Check sheet for the modelled part. Datum: model origin and axes. Units: mm. A direction names the side the tool comes from. Coordinates: 2 decimals unless noted, no trailing zeros. Write each loop counter-clockwise with the first axis right and the second up, starting at its lowest first coordinate (ties: lowest second). Pieces come first, ordered by that corner, then holes. Notation, with made-up numbers: (-11, 78) -> (22, 78) arc R27 cw to (22, 98) -> close; hole circle Ø9 at (80.5, -20). An arc over 180 degrees is marked (long way). One line per item, written item: value. Start each with the question number.
1) Set-up check for faces 1 (the flat face through (3, 98, -222.25)), 2 (the flat face through (3, 165, -90.5)), 3 (the flat face through (3, -4, -209.55)), 4 (the flat face through (3, 0, -251)): record each of +Z, -Z, +X, -X, +Y, -Y from which the full face is reachable in a straight line by a thin tool's end or side.
2) Sectioned sample at B-B on z = -106. Enter the section's corners in (x, y).
3) Scan lines: line 1 along Z through (x, y) = (1.35, 33) (3 decimals); line 2 along Z through (x, y) = (4.45, 175.5); line 3 along Z through (x, y) = (1.85, 20.5). Record each from-to range of solid material in increasing order. Write a range as [from, to].
4) Sectioned sample at C-C on y = 167.5. Enter the section's corners in (x, z).
5) Draft check along Y on faces 5 (the flat face through (3, -7.62, -105)), 6 (the flat face through (3, 31, 0)), 7 (the flat face through (3, 150, -85.471)). Enter one of: +Y half, -Y half, draft (parallel to the pull), parting line (faces both ways), or undercut.
6) Gauge pin test, flat ends, axial feed: P1, Ø1, axis at x = 0.5, z = -50, coming from the +Y side; P2, Ø2, axis at x = 2, z = -87, coming from the -Y side; P3, Ø3, axis at y = 142.5, z = -181.5, coming from the -X side. Record the tip position at first contact, or that the pin passes through.
7) Sectioned sample at A-A on y = 53. Enter the section's corners in (x, z) (3 decimals), plus the area to 3 significant figures.
8) Sectioned sample at D-D on x = 2.5. Give the number of separate pieces and of enclosed holes in the cut face, plus the area to 3 significant figures.
Autodesk Inventor part; units mm, degrees
ref_plane "YZ Plane" through (0, 0, 0) normal (1, 0, 0) x (0, 1, 0)
ref_plane "XZ Plane" through (0, 0, 0) normal (0, 1, 0) x (-1, 0, 0)
ref_plane "XY Plane" through (0, 0, 0) normal (0, 0, 1) x (1, 0, 0)
sketch "Sketch1" plane through (0, 0, 0) normal (1, 0, 0) x (0, 1, 0)
  line L0 (0, 0) -> (177.8, 0)
  line L1 (177.8, -260.35) -> (0, -260.35)
  line L2 (0, -260.35) -> (0, -241.3)
  line L3 (0, -241.3) -> (-7.62, -241.3)
  line L4 (-7.62, -241.3) -> (-7.62, -222.25)
  line L5 (-7.62, -222.25) -> (0, -222.25)
  line L6 (0, -209.55) -> (-7.62, -209.55)
  line L7 (-7.62, -209.55) -> (-7.62, -190.5)
  line L8 (-7.62, -190.5) -> (0, -190.5)
  line L9 (0, -190.5) -> (0, -152.4)
  line L10 (44.45, -215.9) -> (44.45, -214.2998)
  line L11 (44.45, -217.5002) -> (44.45, -215.9)
  line L12 (24.6348, -214.2998) -> (24.6348, -212.725)
  line L13 (24.6348, -219.075) -> (24.6348, -219.329)
  line L14 (24.6348, -219.329) -> (30.1625, -219.329)
  line L15 (24.6348, -212.725) -> (24.6348, -212.471)
  line L16 (24.6348, -212.471) -> (30.1625, -212.471)
  line L17 (24.6348, -219.075) -> (24.6348, -217.4875)
  line L18 (30.1625, -212.471) -> (30.1625, -214.2998)
  line L19 (30.1625, -217.5002) -> (30.1625, -219.329)
  line L20 (44.45, -214.2998) -> (30.1625, -214.2998)
  line L21 (24.6348, -214.2998) -> (0, -214.2998)
  line L22 (44.45, -217.5002) -> (30.1625, -217.5002)
  line L23 (24.6348, -217.5002) -> (0, -217.5002)
  line L24 (0, -63.5) -> (-7.62, -63.5)
  line L25 (-7.62, -63.5) -> (-7.62, -82.55)
  line L26 (-7.62, -82.55) -> (0, -82.55)
  line L27 (0, -95.25) -> (-7.62, -95.25)
  line L28 (-7.62, -95.25) -> (-7.62, -114.3)
  line L29 (-7.62, -114.3) -> (0, -114.3)
  line L30 (44.45, -88.9) -> (44.45, -90.5002)
  line L31 (44.45, -87.2998) -> (44.45, -88.9)
  line L32 (24.6348, -90.5002) -> (24.6348, -92.075)
  line L33 (24.6348, -85.725) -> (24.6348, -85.471)
  line L34 (24.6348, -85.471) -> (30.1625, -85.471)
  line L35 (24.6348, -92.075) -> (24.6348, -92.329)
  line L36 (24.6348, -92.329) -> (30.1625, -92.329)
  line L37 (24.6348, -85.725) -> (24.6348, -87.3125)
  line L38 (30.1625, -92.329) -> (30.1625, -90.5002)
  line L39 (30.1625, -87.2998) -> (30.1625, -85.471)
  line L40 (44.45, -90.5002) -> (30.1625, -90.5002)
  line L41 (24.6348, -90.5002) -> (0, -90.5002)
  line L42 (44.45, -87.2998) -> (30.1625, -87.2998)
  line L43 (24.6348, -87.2998) -> (0, -87.2998)
  line L44 (177.8, -241.3) -> (185.42, -241.3)
  line L45 (185.42, -241.3) -> (185.42, -222.25)
  line L46 (185.42, -222.25) -> (177.8, -222.25)
  line L47 (177.8, -209.55) -> (185.42, -209.55)
  line L48 (185.42, -209.55) -> (185.42, -190.5)
  line L49 (185.42, -190.5) -> (177.8, -190.5)
  line L50 (177.8, -190.5) -> (177.8, -152.4)
  line L51 (133.35, -215.9) -> (133.35, -214.2998)
  line L52 (133.35, -217.5002) -> (133.35, -215.9)
  line L53 (153.1652, -214.2998) -> (153.1652, -212.725)
  line L54 (153.1652, -219.075) -> (153.1652, -219.329)
  line L55 (153.1652, -219.329) -> (147.6375, -219.329)
  line L56 (153.1652, -212.725) -> (153.1652, -212.471)
  line L57 (153.1652, -212.471) -> (147.6375, -212.471)
  line L58 (153.1652, -219.075) -> (153.1652, -217.4875)
  line L59 (147.6375, -212.471) -> (147.6375, -214.2998)
  line L60 (147.6375, -217.5002) -> (147.6375, -219.329)
  line L61 (133.35, -214.2998) -> (147.6375, -214.2998)
  line L62 (153.1652, -214.2998) -> (177.8, -214.2998)
  line L63 (133.35, -217.5002) -> (147.6375, -217.5002)
  line L64 (153.1652, -217.5002) -> (177.8, -217.5002)
  line L65 (185.42, -63.5) -> (185.42, -82.55)
  line L66 (185.42, -82.55) -> (177.8, -82.55)
  line L67 (177.8, -95.25) -> (185.42, -95.25)
  line L68 (185.42, -95.25) -> (185.42, -114.3)
  line L69 (185.42, -114.3) -> (177.8, -114.3)
  line L70 (153.1652, -85.725) -> (153.1652, -85.471)
  line L71 (153.1652, -85.725) -> (153.1652, -87.3125)
  line L72 (153.1652, -85.471) -> (147.6375, -85.471)
  line L73 (147.6375, -87.2998) -> (147.6375, -85.471)
  line L74 (177.8, -63.5) -> (185.42, -63.5)
  line L75 (153.1652, -90.5002) -> (153.1652, -92.075)
  line L76 (153.1652, -92.075) -> (153.1652, -92.329)
  line L77 (153.1652, -92.329) -> (147.6375, -92.329)
  line L78 (147.6375, -92.329) -> (147.6375, -90.5002)
  line L79 (133.35, -87.2998) -> (147.6375, -87.2998)
  line L80 (133.35, -87.2998) -> (133.35, -88.9)
  line L81 (133.35, -90.5002) -> (147.6375, -90.5002)
  line L82 (153.1652, -87.2998) -> (177.8, -87.2998)
  line L83 (153.1652, -90.5002) -> (177.8, -90.5002)
  line L84 (133.35, -88.9) -> (133.35, -90.5002)
  line L85 (177.8, -260.35) -> (177.8, -254)
  line L86 (177.8, -254) -> (88.9, -254)
  line L87 (88.9, -254) -> (88.9, -247.65)
  line L88 (88.9, -247.65) -> (177.8, -247.65)
  line L89 (177.8, -254) -> (177.8, -260.35)
  line L90 (177.8, 0) -> (177.8, -63.5)
  line L91 (177.8, -114.3) -> (177.8, -190.5)
  line L92 (177.8, -241.3) -> (177.8, -247.65)
  line L93 (0, -260.35) -> (0, -241.3)
  line L94 (0, -190.5) -> (0, -114.3)
  line L95 (0, -63.5) -> (0, 0)
  line L96 (0, -82.55) -> (0, -87.2998)
  line L97 (0, -90.5002) -> (0, -95.25)
  line L98 (0, -95.25) -> (0, -90.5002)
  line L99 (0, -87.2998) -> (0, -82.55)
  line L100 (0, -222.25) -> (0, -217.5002)
  line L101 (0, -214.2998) -> (0, -209.55)
  line L102 (0, -222.25) -> (0, -217.5002)
  line L103 (0, -214.2998) -> (0, -209.55)
  line L104 (177.8, -222.25) -> (177.8, -217.5002)
  line L105 (177.8, -214.2998) -> (177.8, -209.55)
  line L106 (177.8, -209.55) -> (177.8, -214.2998)
  line L107 (177.8, -217.5002) -> (177.8, -222.25)
  line L108 (177.8, -82.55) -> (177.8, -87.2998)
  line L109 (177.8, -90.5002) -> (177.8, -95.25)
  line L110 (177.8, -82.55) -> (177.8, -87.2998)
  line L111 (177.8, -90.5002) -> (177.8, -95.25)
  dimension "d0" = 177.8
  dimension "d1" = 260.35
  dimension "d8" = 38.1
  dimension "d16" = 0.254
  dimension "d17" = 0.254
  dimension "d18" = 6.35
extrude "Extrusion1" add sketch "Sketch1" along normal blind 5.5563
sketch "Sketch2" plane through (5.5563, 0, 0) normal (1, 0, 0) x (0, 0, -1)
  line L0 (63.5, 177.8) -> (0, 177.8)
  line L1 (0, 177.8) -> (50.8, 177.8)
  line L2 (50.8, 177.8) -> (50.8, 63.5)
  line L3 (50.8, 63.5) -> (0, 63.5)
  line L4 (0, 177.8) -> (0, 0)
  line L5 (0, 177.8) -> (0, 63.5)
extrude "Extrusion2" cut sketch "Sketch2" against normal blind 25.4
sketch "Sketch3" plane through (5.5563, 0, 0) normal (1, 0, 0) x (0, 0, -1)
  line L0 (190.5, 177.8) -> (114.3, 177.8)
  line L1 (247.65, 88.9) -> (247.65, 177.8)
  line L2 (76.2, 100.8) -> (76.2, 95.25)
  line L3 (114.3, 95.25) -> (114.3, 100.8)
  line L4 (184.15, 100.8) -> (184.15, 95.25)
  line L5 (222.25, 95.25) -> (222.25, 100.8)
  line L6 (76.2, 100.8) -> (114.3, 100.8)
  line L7 (184.15, 100.8) -> (222.25, 100.8)
  line L8 (95.25, 95.25) -> (76.2, 95.25)
  line L9 (95.25, 95.25) -> (114.3, 95.25)
  line L10 (184.15, 95.25) -> (222.25, 95.25)
  point P0 (0, 0)
extrude "Extrusion3" cut sketch "Sketch3" against normal blind 25.4
sketch "Sketch4" plane through (5.5563, 0, 0) normal (1, 0, 0) x (0, 0, -1)
  line L0 (111.9187, 28.194) -> (117.475, 28.194)
  line L1 (117.475, 28.194) -> (117.475, 66.294)
  line L2 (117.475, 66.294) -> (111.9187, 66.294)
  line L3 (111.9187, 47.244) -> (111.9187, 66.294)
  line L4 (111.9187, 28.194) -> (111.9187, 47.244)
  point P0 (0, 0)
extrude "Extrusion4" cut sketch "Sketch4" against normal blind 25.4
properties part number "sidewall"
Answers:
1. face 1: +X, -X
1. face 2: +X, -X, +Y
1. face 3: +X, -X, -Y
1. face 4: -Z, +X, -X, -Y
2. outline: (0, -7.62) -> (5.56, -7.62) -> (5.56, 95.25) -> (0, 95.25) -> close; (0, 100.8) -> (5.56, 100.8) -> (5.56, 185.42) -> (0, 185.42) -> close
3. line 1: z = [-260.35, -217.5], [-214.3, -117.475], [-111.919, -90.5], [-87.3, 0]
3. line 2: z = [-260.35, -254], [-247.65, -217.5], [-214.3, -90.5], [-87.3, -50.8]
3. line 3: z = [-260.35, -217.5], [-214.3, -90.5], [-87.3, 0]
4. outline: (0, -260.35) -> (5.56, -260.35) -> (5.56, -254) -> (0, -254) -> close; (0, -247.65) -> (5.56, -247.65) -> (5.56, -217.5) -> (0, -217.5) -> close; (0, -214.3) -> (5.56, -214.3) -> (5.56, -90.5) -> (0, -90.5) -> close; (0, -87.3) -> (5.56, -87.3) -> (5.56, -50.8) -> (0, -50.8) -> close
5. face 5: -Y half
5. face 6: draft
5. face 7: undercut
6. P1: stops at y = 63.5
6. P2: stops at y = 0
6. P3: stops at x = 0
7. outline: (0, -260.35) -> (5.556, -260.35) -> (5.556, -117.475) -> (0, -117.475) -> close; (0, -111.919) -> (5.556, -111.919) -> (5.556, 0) -> (0, 0) -> close
7. area: 1,420 mm2
8. separate pieces: 1
8. enclosed holes: 3
8. area: 39,800 mm2
